```python
from build123d import *

# Parameters (mm, degrees)
ESBO_O1_W                                         = 25
ESBO_O1_H                                         = 25
RESSALTO_EXTRUS_O1_DEPTH                          = 40
ESBO_O2_R                                         = 5.1
CORTE_EXTRUS_O1_DEPTH                             = 41
ESBO_O3_R                                         = 11
CORTE_EXTRUS_O2_DEPTH                             = 3.2
FURO_ROSCADO_PARA_CONDU_TE_DE_M3X0_52_D           = 3.15
FURO_ROSCADO_PARA_CONDU_TE_DE_M3X0_52_DEPTH       = 6
FURO_ROSCADO_PARA_CONDU_TE_DE_M3X0_52_CSINK_D     = 3.766
FURO_ROSCADO_PARA_CONDU_TE_DE_M3X0_52_CSINK_ANGLE = 90
FURO_ROSCADO_PARA_CONDU_TE_DE_M3X0_52_TIP         = 0.946355475
REBAIXO_PARA_SHCS_M31_AT_2_COUNT                  = 2
REBAIXO_PARA_SHCS_M31_AT_2_PITCH                  = 16
REBAIXO_PARA_SHCS_M31_AT_3_COUNT                  = 2
REBAIXO_PARA_SHCS_M31_AT_3_PITCH                  = 16
REBAIXO_PARA_SHCS_M31_AT_4_COUNT                  = 2
REBAIXO_PARA_SHCS_M31_AT_4_PITCH                  = 22.627416998
FURO_ROSCADO_PARA_CONDU_TE_DE_M3X0_53_D           = 3.15
FURO_ROSCADO_PARA_CONDU_TE_DE_M3X0_53_DEPTH       = 8
FURO_ROSCADO_PARA_CONDU_TE_DE_M3X0_53_CSINK_D     = 3.766
FURO_ROSCADO_PARA_CONDU_TE_DE_M3X0_53_CSINK_ANGLE = 90
FURO_ROSCADO_PARA_CONDU_TE_DE_M3X0_53_TIP         = 0.946355475


with BuildPart() as part:
    # Esboço1 → Ressalto-extrusão1 (new body)
    with BuildSketch(Plane.XY):
        Rectangle(ESBO_O1_W, ESBO_O1_H)
    extrude(amount=RESSALTO_EXTRUS_O1_DEPTH)

    # Esboço2 → Corte-extrusão1 (cut, through all)
    with BuildSketch(Plane.XY.offset(40)):
        Circle(ESBO_O2_R)
    extrude(amount=-CORTE_EXTRUS_O1_DEPTH, mode=Mode.SUBTRACT)

    # Esboço3 → Corte-extrusão2 (cut)
    with BuildSketch(Plane.XY.offset(40)):
        Circle(ESBO_O3_R)
    extrude(amount=-CORTE_EXTRUS_O2_DEPTH, mode=Mode.SUBTRACT)

    # Furo roscado para conduíte de M3x0.52
    with Locations(Plane.XY.offset(36.8)):
        with Locations((0, 8), (8, 0), (0, -8), (-8, 0)):
            CounterSinkHole(FURO_ROSCADO_PARA_CONDU_TE_DE_M3X0_52_D / 2, FURO_ROSCADO_PARA_CONDU_TE_DE_M3X0_52_CSINK_D / 2, depth=FURO_ROSCADO_PARA_CONDU_TE_DE_M3X0_52_DEPTH, counter_sink_angle=FURO_ROSCADO_PARA_CONDU_TE_DE_M3X0_52_CSINK_ANGLE)
            with Locations((0, 0, -(FURO_ROSCADO_PARA_CONDU_TE_DE_M3X0_52_DEPTH + FURO_ROSCADO_PARA_CONDU_TE_DE_M3X0_52_TIP / 2))):  # 118° drill point
                Cone(0, FURO_ROSCADO_PARA_CONDU_TE_DE_M3X0_52_D / 2, FURO_ROSCADO_PARA_CONDU_TE_DE_M3X0_52_TIP, mode=Mode.SUBTRACT)

    # Esboço13 → Rebaixo para SHCS M31 (revolve, cut)
    with BuildSketch(Plane(origin=(-8, 12.5, 12), x_dir=(0, 0, 1), z_dir=(1, 0, 0))):
        Polygon((0, 0), (0, 25), (1.7, 25), (1.7, 3), (3.25, 3), (3.25, 0.025), (3.275, 0), align=None)
    rebaixo_para_shcs_m31 = revolve(axis=Axis((-8, 18.85, 12), (0, -1, 0)), mode=Mode.SUBTRACT)

    # Rebaixo para SHCS M31 at 2: Rebaixo para SHCS M31 ×2
    with Locations(*[(i * REBAIXO_PARA_SHCS_M31_AT_2_PITCH, 0, 0) for i in range(1, REBAIXO_PARA_SHCS_M31_AT_2_COUNT)]):
        add(rebaixo_para_shcs_m31, mode=Mode.SUBTRACT)

    # Rebaixo para SHCS M31 at 3: Rebaixo para SHCS M31 ×2
    with Locations(*[(0, 0, i * REBAIXO_PARA_SHCS_M31_AT_3_PITCH) for i in range(1, REBAIXO_PARA_SHCS_M31_AT_3_COUNT)]):
        add(rebaixo_para_shcs_m31, mode=Mode.SUBTRACT)

    # Rebaixo para SHCS M31 at 4: Rebaixo para SHCS M31 ×2
    with Locations(*[Vector(0.707106781, 0, 0.707106781) * (i * REBAIXO_PARA_SHCS_M31_AT_4_PITCH) for i in range(1, REBAIXO_PARA_SHCS_M31_AT_4_COUNT)]):
        add(rebaixo_para_shcs_m31, mode=Mode.SUBTRACT)

    # Furo roscado para conduíte de M3x0.53
    with Locations(Plane(origin=(0, 12.5, 0), x_dir=(1, 0, 0), z_dir=(0, 1, 0))):
        with Locations((-8, -5), (8, -5), (-8, -35), (8, -35)):
            CounterSinkHole(FURO_ROSCADO_PARA_CONDU_TE_DE_M3X0_53_D / 2, FURO_ROSCADO_PARA_CONDU_TE_DE_M3X0_53_CSINK_D / 2, depth=FURO_ROSCADO_PARA_CONDU_TE_DE_M3X0_53_DEPTH, counter_sink_angle=FURO_ROSCADO_PARA_CONDU_TE_DE_M3X0_53_CSINK_ANGLE)
            with Locations((0, 0, -(FURO_ROSCADO_PARA_CONDU_TE_DE_M3X0_53_DEPTH + FURO_ROSCADO_PARA_CONDU_TE_DE_M3X0_53_TIP / 2))):  # 118° drill point
                Cone(0, FURO_ROSCADO_PARA_CONDU_TE_DE_M3X0_53_D / 2, FURO_ROSCADO_PARA_CONDU_TE_DE_M3X0_53_TIP, mode=Mode.SUBTRACT)


solid = part.part
```
Could you check a few things on this model? Use its own coordinates, in mm. A direction names the side the tool comes from. Round coordinates to 2 decimals unless told otherwise and drop trailing zeros. Write each loop counter-clockwise with the first axis right and the second up, starting at its lowest first coordinate (ties: lowest second). Pieces come first, ordered by that corner, then holes.
(1) If I drill on probe 1 along Z at (x, y) = (8, -4.5); probe 2 along X at (y, z) = (8.5, 5) (3 decimals); probe 3 along Y at (x, z) = (0, 32.25) (3 decimals), over which ranges is the centre line in solid material (lowest first)?
Findings below:
probe 1: z = 0 to 10.3, 13.7 to 26.3, 29.7 to 36.8
probe 2: x = -12.5 to -9.575, -6.425 to 6.425, 9.575 to 12.5
probe 3: y = -12.5 to -9.575, -6.425 to -5.1, 5.1 to 6.425, 9.575 to 12.5
(2) For pin 1 (12 mm diameter, centred on x = 9, y = -5, fed in from -Z); pin 2 (2 mm diameter, centred on x = 8, z = 13, fed in from +Y); pin 3 (2 mm diameter, centred on x = -8, z = 28, fed in from -Y); pin 4 (1.9 mm diameter, centred on x = 0, y = -8, fed in from +Z), each with a flat end and sliding along its axis, tell me the tip position at first contact or that it passes through.
Findings below:
pin 1: stops at z = 0
pin 2: stops at y = 9.5
pin 3: passes through
pin 4: stops at z = 30.42
(3) Suppose I cut it at C-C on y = 9. State how many separate pieces and enclosed holes the cut face has, and give its area (3 significant figures).
Findings below:
separate pieces: 1
enclosed holes: 8
area: 877 mm2
(4) Thinking about a two-plate mould opening in Z: for faces 4 (the face through (9.4, 9.5, 26.6)), 5 (the face through (0.21, -6.44, 33.61)), 6 (the face through (-8.273, 0.012, 30.018)), which applies, +Z half, -Z half, draft (parallel to the pull), parting line (faces both ways), or undercut?
Findings below:
face 4: undercut
face 5: draft
face 6: +Z half
(5) Suppose I cut it at B-B on z = 17.5. Write out the boundary of the cut face in (x, y), and give its area (3 significant figures).
Findings below:
outline: (-12.5, -12.5) - (12.5, -12.5) - (12.5, 12.5) - (-12.5, 12.5) - close; hole circle Ø10.2 at (0, 0)
area: 543 mm2
(6) Suppose I cut it at A-A on z = 28. Write out the boundary of the cut face in (x, y) (3 decimals).
Findings below:
outline: (-12.5, -12.5) - (-9.7, -12.5) - (-9.7, 9.5) - (-11.25, 9.5) - (-11.25, 12.475) - (-11.275, 12.5) - (-12.5, 12.5) - close; (-6.3, -12.5) - (6.3, -12.5) - (6.3, 9.5) - (4.75, 9.5) - (4.75, 12.475) - (4.725, 12.5) - (-4.725, 12.5) - (-4.75, 12.475) - (-4.75, 9.5) - (-6.3, 9.5) - close; (9.7, -12.5) - (12.5, -12.5) - (12.5, 12.5) - (11.275, 12.5) - (11.25, 12.475) - (11.25, 9.5) - (9.7, 9.5) - close; hole circle Ø10.2 at (0, 0)
(7) Which directions (+Z, -Z, +X, -X, +Y, -Y) give clear straight access to the entire face, cutting with the end or side of a thin tool? Please do faces 1 (the face through (-10.197, 11.008, 9.605)), 2 (the face through (0.341, 6.462, 33.606)), 3 (the face through (9.03, -1.35, 26.65)).
Findings below:
face 1: +Y
face 2: +Z
face 3: +Y, -Y
